```python
from build123d import *

# Parameters (mm, degrees)
F0_W     = 26
F0_H     = 24
F0_R     = 1.15
F0_R_2   = 2.15
F1_DEPTH = 3
F2_W     = 7
F2_H     = 5
F3_DEPTH = 2
F4_R     = 2


with BuildPart() as f1:
    # F0 (on Top) → F1 (new body)
    with BuildSketch(Plane.XY):
        with Locations((13, -12)):
            Rectangle(F0_W, F0_H)
        with Locations((5, -19)):
            Circle(F0_R, mode=Mode.SUBTRACT)
        with Locations((14.5, -19)):
            Circle(F0_R, mode=Mode.SUBTRACT)
        with Locations((8, -10)):
            Circle(F0_R_2, mode=Mode.SUBTRACT)
    extrude(amount=F1_DEPTH)

    # F2 (on face) → F3 (join)
    with BuildSketch(Plane.XY.offset(3)):
        with Locations((22.5, -10)):
            Rectangle(F2_W, F2_H)
    extrude(amount=F3_DEPTH)

    # F4
    f4_edges = [f1.edges().sort_by_distance(p)[0] for p in [
        (0, -24, 1.5),
        (26, -24, 1.5),
    ]]
    fillet(f4_edges, radius=F4_R)


solid = f1.part
```
The listing builds one solid part. Answer for the finished solid, in the listing's coordinates (mm). A direction names the side the tool comes from. Coordinates: 2 decimals unless noted, no trailing zeros. Order: outer loops, then holes, each group sorted by start corner. A loop starts at its lowest first (then second) coordinate and runs counter-clockwise, first axis right, second up. Notation, with made-up numbers: M 7.5,63 L 15.5,63 A38 ccw 15.5,102 Z; hole C -27,-24.75 d8. An arc over 180 degrees is marked long. Answer as a JSON object with one key per item and string values. Group by question number.
1. Determine the mould class of faces 4 (the cylindrical face through (13.59, -19.7, 1.48)), 5 (the cylindrical face through (9.16, -8.19, 1.48)), 6 (the cylindrical face through (25.4, -23.43, 1.52)), 7 (the flat face through (22, -7.5, 4)) for opening direction Y: released by +Y, released by -Y, zero draft, split by the parting line, or undercut.
2. A tool of negligible diameter and unlimited length cuts with its end or side. For faces 1 (the flat face through (22, -12.5, 4)), 2 (the cylindrical face through (4.09, -19.7, 1.48)), 3 (the flat face through (19, -10, 4)), from which of +Z, -Z, +X, -X, +Y, -Y can it reach the whole face along a straight path? Write none if from no direction.
3. Section B-B on x = 5 is taken. Write down the section's boundary in (y, z), then the cut area to 3 significant figures.
4. Flat-ended cylindrical pins translate along their axes: P1, Ø2, axis at y = -10.5, z = 4.5, coming from the -X side; P2, Ø1.8, axis at x = 5, y = -19, coming from the +Z side. Find the tip coordinate at first contact, or state that the pin passes through.
5. Section D-D on x = 8 is taken. Write down the section's boundary in (y, z).
6. Section A-A on y = -10 is taken. Write down the section's boundary in (x, z), then the cut area to 3 significant figures.
7. Section C-C on z = 0.3 is taken. Write down the section's boundary in (x, y), then the cut area to 3 significant figures.
8. Straight lines are drawn through the part: line 1 (Y direction, x = 14.5, z = 0.9); line 2 (Y direction, x = 8, z = 0.75); line 3 (X direction, y = -19.5, z = 2.1). For each, find the intervals that lie inside material, in ascending order.
Values follow:
{
 "1": {"face 4": "undercut", "face 5": "undercut", "face 6": "released by -Y", "face 7": "released by +Y"},
 "2": {"face 1": "+Z, +X, -X, -Y", "face 2": "+Z, -Z", "face 3": "+Z, -X, +Y, -Y"},
 "3": {"outline": "M -24,0 L -20.15,0 L -20.15,3 L -24,3 Z; M -17.85,0 L 0,0 L 0,3 L -17.85,3 Z", "area": "65.1 mm2"},
 "4": {"P1": "x = 19", "P2": "through"},
 "5": {"outline": "M -24,0 L -12.15,0 L -12.15,3 L -24,3 Z; M -7.85,0 L 0,0 L 0,3 L -7.85,3 Z"},
 "6": {"outline": "M 0,0 L 5.85,0 L 5.85,3 L 0,3 Z; M 10.15,0 L 26,0 L 26,5 L 19,5 L 19,3 L 10.15,3 Z", "area": "79.1 mm2"},
 "7": {"outline": "M 0,-22 A2 ccw 2,-24 L 24,-24 A2 ccw 26,-22 L 26,0 L 0,0 Z; hole C 5,-19 d2.3; hole C 8,-10 d4.3; hole C 14.5,-19 d2.3", "area": "599 mm2"},
 "8": {"line 1": "-24 to -20.15, -17.85 to 0", "line 2": "-24 to -12.15, -7.85 to 0", "line 3": "0 to 3.96, 6.04 to 13.46, 15.54 to 26"}
}
